```python
from build123d import *

# Parameters (mm, degrees)
BOSS_EXTRUDE1_DEPTH                                 = 70
BOSS_EXTRUDE2_REACH                                 = 115.806
BOSS_EXTRUDE2_START_RADIUS                          = 57
BOSS_EXTRUDE2_END_RADIUS                            = 57
SKETCH7_W                                           = 3
SKETCH7_H                                           = 10
CSK_FOR_M4_COUNTERSUNK_FLAT_HEAD_SCREW2_D           = 4.5
CSK_FOR_M4_COUNTERSUNK_FLAT_HEAD_SCREW2_DEPTH       = 11.5
CSK_FOR_M4_COUNTERSUNK_FLAT_HEAD_SCREW2_CSINK_D     = 9.4
CSK_FOR_M4_COUNTERSUNK_FLAT_HEAD_SCREW2_CSINK_ANGLE = 90
CSK_FOR_M4_COUNTERSUNK_FLAT_HEAD_SCREW2_TIP         = 1.351936393
FILLET1_R                                           = 10


with BuildPart() as part:
    # Sketch2 → Boss-Extrude1 (new, symmetric)
    with BuildSketch(Plane(origin=(0, 0, 0), x_dir=(1, 0, 0), z_dir=(0, 1, 0))):
        with BuildLine():
            Line((-47.704446333, -36.390737834), (-45.562994128, -34.249285629))
            ThreePointArc((-45.562994128, -34.249285629), (0, -57), (45.562994128, -34.249285629))
            Line((45.562994128, -34.249285629), (47.704446333, -36.390737834))
            ThreePointArc((47.704446333, -36.390737834), (0, -60), (-47.704446333, -36.390737834))
        make_face()
    extrude(amount=BOSS_EXTRUDE1_DEPTH, both=True)

    # Boss-Extrude2: from a cylinder face, 115.806 long prism both ways, kept between that surface and its translate by the depth
    boss_extrude2_start = Plane(origin=(0, 0.207736, 0), z_dir=(0, -1, 0)) * Cylinder(BOSS_EXTRUDE2_START_RADIUS, 477.027472, mode=Mode.PRIVATE)
    boss_extrude2_end = Plane(origin=(0, 0.207736, -10), z_dir=(0, -1, 0)) * Cylinder(BOSS_EXTRUDE2_END_RADIUS, 477.027472, mode=Mode.PRIVATE)
    # Sketch7 → Boss-Extrude2 (add, from a surface)
    with BuildSketch(Plane.XY, mode=Mode.PRIVATE) as boss_extrude2_sk1:
        with Locations((4.5, -65)):
            Rectangle(SKETCH7_W, SKETCH7_H)
    boss_extrude2_tool1 = extrude(boss_extrude2_sk1.sketch, amount=BOSS_EXTRUDE2_REACH, both=True, mode=Mode.PRIVATE)
    add(((boss_extrude2_tool1 & boss_extrude2_start) - boss_extrude2_end).solids().sort_by_distance((4.5, -65, 51.802164))[0])
    # Sketch7 → Boss-Extrude2 (add, from a surface)
    with BuildSketch(Plane.XY, mode=Mode.PRIVATE) as boss_extrude2_sk2:
        with BuildLine():
            Line((3, 65.553629026), (3, 64))
            Line((3, 64), (6, 64))
            Line((6, 64), (6, 67.370437785))
            Line((6, 67.370437785), (3.649292783, 66.490114182))
            ThreePointArc((3.649292783, 66.490114182), (3.178200993, 66.123406518), (3, 65.553629026))
        make_face()
    boss_extrude2_tool2 = extrude(boss_extrude2_sk2.sketch, amount=BOSS_EXTRUDE2_REACH, both=True, mode=Mode.PRIVATE)
    add(((boss_extrude2_tool2 & boss_extrude2_start) - boss_extrude2_end).solids().sort_by_distance((4.5, -65, 51.802164))[0])
    # Sketch7 → Boss-Extrude2 (add, from a surface)
    with BuildSketch(Plane.XY, mode=Mode.PRIVATE) as boss_extrude2_sk3:
        with BuildLine():
            Line((-3, 65.553629026), (-3, 64))
            Line((-3, 64), (-6, 64))
            Line((-6, 64), (-6, 67.370437785))
            Line((-6, 67.370437785), (-3.649292783, 66.490114182))
            ThreePointArc((-3.649292783, 66.490114182), (-3.178200993, 66.123406518), (-3, 65.553629026))
        make_face()
    boss_extrude2_tool3 = extrude(boss_extrude2_sk3.sketch, amount=BOSS_EXTRUDE2_REACH, both=True, mode=Mode.PRIVATE)
    add(((boss_extrude2_tool3 & boss_extrude2_start) - boss_extrude2_end).solids().sort_by_distance((4.5, -65, 51.802164))[0])
    # Sketch7 → Boss-Extrude2 (add, from a surface)
    with BuildSketch(Plane.XY, mode=Mode.PRIVATE) as boss_extrude2_sk4:
        with Locations((-4.5, -65)):
            Rectangle(SKETCH7_W, SKETCH7_H)
    boss_extrude2_tool4 = extrude(boss_extrude2_sk4.sketch, amount=BOSS_EXTRUDE2_REACH, both=True, mode=Mode.PRIVATE)
    add(((boss_extrude2_tool4 & boss_extrude2_start) - boss_extrude2_end).solids().sort_by_distance((4.5, -65, 51.802164))[0])

    # CSK for M4 Countersunk Flat Head Screw2
    with Locations(Plane(origin=(0, 55, 60), x_dir=(1, 0, 0), z_dir=(0, 0, 1))):
        with Locations((0, 0), (0, -110)):
            CounterSinkHole(CSK_FOR_M4_COUNTERSUNK_FLAT_HEAD_SCREW2_D / 2, CSK_FOR_M4_COUNTERSUNK_FLAT_HEAD_SCREW2_CSINK_D / 2, depth=CSK_FOR_M4_COUNTERSUNK_FLAT_HEAD_SCREW2_DEPTH, counter_sink_angle=CSK_FOR_M4_COUNTERSUNK_FLAT_HEAD_SCREW2_CSINK_ANGLE)
            with Locations((0, 0, -(CSK_FOR_M4_COUNTERSUNK_FLAT_HEAD_SCREW2_DEPTH + CSK_FOR_M4_COUNTERSUNK_FLAT_HEAD_SCREW2_TIP / 2))):  # 118° drill point
                Cone(0, CSK_FOR_M4_COUNTERSUNK_FLAT_HEAD_SCREW2_D / 2, CSK_FOR_M4_COUNTERSUNK_FLAT_HEAD_SCREW2_TIP, mode=Mode.SUBTRACT)

    # Fillet1
    fillet1_edges = [part.edges().sort_by_distance(p)[0] for p in [
        (-46.63372023, 70, 35.320011731),
        (-46.63372023, -70, 35.320011731),
        (46.63372023, -70, 35.320011731),
        (46.63372023, 70, 35.320011731),
    ]]
    fillet(fillet1_edges, radius=FILLET1_R)


solid = part.part
```
The model under review builds one solid part; all positions refer to its coordinate system, in mm. A direction names the side the tool comes from. Give positions to 0.01 mm unless a question says otherwise; leave off trailing zeros. Write each loop counter-clockwise with the first axis right and the second up, starting at its lowest first coordinate (ties: lowest second). Pieces come first, ordered by that corner, then holes. Notation, with made-up numbers: (-38, 75) -> (17, 75) arc R10 ccw to (17, 89) -> close; hole circle Ø11 at (-14, 60). An arc over 180 degrees is marked (long way). Answer in a Markdown table with one row per item.
1) Mouldability with a two-part tool opening along Y and no side actions: class faces 1 (the flat face through (3.2, -70, 52.2)), 2 (the flat face through (-3, -65, 52)), 3 (the flat face through (-5, -60, 52)) as +Y half, -Y half, draft (parallel to the pull), parting line (faces both ways), or undercut.
Worked answers:
| item | result |
|---|---|
| face 1 | -Y half |
| face 2 | draft |
| face 3 | undercut |
2) Add section A-A on x = 0. State the section outline as (y, z) points, plus the area to 3 significant figures.
Worked answers:
| item | result |
|---|---|
| outline | (-70, 57) -> (-57.25, 57) -> (-57.25, 57.55) -> (-59.7, 60) -> (-70, 60) -> close; (-52.75, 57) -> (52.75, 57) -> (52.75, 57.55) -> (50.3, 60) -> (-50.3, 60) -> (-52.75, 57.55) -> close; (57.25, 57) -> (70, 57) -> (70, 60) -> (59.7, 60) -> (57.25, 57.55) -> close |
| area | 381 mm² |
3) Add section C-C on z = 51.25. State the section outline as (x, y) points.
Worked answers:
| item | result |
|---|---|
| outline | (-31.2, -70) -> (-24.95, -70) -> (-24.95, 70) -> (-31.2, 70) -> close; (-6, -70) -> (-3, -70) -> (-3, -60) -> (-6, -60) -> close; (-6, 64) -> (-3, 64) -> (-3, 65.55) arc R1 ccw to (-3.65, 66.49) -> (-6, 67.37) -> close; (3, -70) -> (6, -70) -> (6, -60) -> (3, -60) -> close; (3, 64) -> (6, 64) -> (6, 67.37) -> (3.65, 66.49) arc R1 ccw to (3, 65.55) -> close; (24.95, -70) -> (31.2, -70) -> (31.2, 70) -> (24.95, 70) -> close |
4) Add section D-D on y = -30. State the section outline as (x, z) points.
Worked answers:
| item | result |
|---|---|
| outline | (-47.7, 36.39) -> (-45.56, 34.25) arc R57 cw to (45.56, 34.25) -> (47.7, 36.39) arc R60 ccw to start |
5) Clearance check with flat-ended pins moving along their axes: P1, Ø0.9, axis at x = 5, z = 53.5, coming from the +Y side; P2, Ø1.2, axis at y = 64.5, z = 52, coming from the -X side; P3, Ø2.5, axis at y = 65, z = 54, coming from the +X side; P4, Ø8, axis at x = 30.5, z = 52.5, coming from the +Y side. State where each tip first meets the part, or that it passes through.
Worked answers:
| item | result |
|---|---|
| P1 | y = 67.16 |
| P2 | x = -30.95 |
| P3 | x = 28.59 |
| P4 | y = 70 |
6) For L1, parallel to Y at x = 0, z = 57.3; L2, parallel to X at y = 46, z = 49.75; L3, parallel to X at y = 43, z = 47.75, list the stretches that pass through material, from the lowest coordinate up. Write a range as [from, to].
Worked answers:
| item | result |
|---|---|
| L1 | [-70, -57.25], [-52.75, 52.75], [57.25, 70] |
| L2 | [-33.54, -27.82], [27.82, 33.54] |
| L3 | [-36.33, -31.13], [31.13, 36.33] |
7) Tool access review of faces 4 (the flat face through (-6, 66, 52)), 5 (the cylindrical face through (0.772, 0.98, 59.995)), 6 (the flat face through (-4, 64, 52)): name each direction out of +Z, -Z, +X, -X, +Y, -Y from which nothing blocks a thin tool from reaching the whole face with its end or side.
Worked answers:
| item | result |
|---|---|
| face 4 | -Z, +Y, -Y |
| face 5 | +Z, +Y, -Y |
| face 6 | -Z |
8) Add section B-B on y = 55. State the section outline as (x, z) points.
Worked answers:
| item | result |
|---|---|
| outline | (-47.7, 36.39) -> (-45.56, 34.25) arc R57 cw to (-2.25, 56.96) -> (-2.25, 57.55) -> (-4.53, 59.83) arc R60 ccw to start; (2.25, 56.96) arc R57 cw to (45.56, 34.25) -> (47.7, 36.39) arc R60 ccw to (4.53, 59.83) -> (2.25, 57.55) -> close |
